Build history of the part. All positions in model axes, mm. A direction names the side the tool comes from. Coordinates: 2 decimals unless noted, no trailing zeros. Loops run counter-clockwise (first coordinate to the right, second up) from the corner with the lowest first, then second, coordinate; pieces in that order, holes last. Notation, with made-up numbers: (55, 89) -> (85, 89) arc R27 cw to (85, 113) -> close; hole circle Ø4 at (69.25, 14.5). An arc over 180 degrees is marked (long way). One line per item, written item: value. Start each with the question number.
Autodesk Inventor part; units mm, degrees
ref_plane "YZ Plane" through (0, 0, 0) normal (1, 0, 0) x (0, 1, 0)
ref_plane "XZ Plane" through (0, 0, 0) normal (0, 1, 0) x (-1, 0, 0)
ref_plane "XY Plane" through (0, 0, 0) normal (0, 0, 1) x (1, 0, 0)
sketch "Esboço1" plane through (0, 0, 0) normal (0, 0, 1) x (1, 0, 0)
  circle A0 centre (0, 0) radius 9
  circle A1 centre (0, 0) radius 11
  point P0 (0, 0)
  dimension "d0" = 2
extrude "Extrusão1" add sketch "Esboço1" along normal blind 5 contours A0 | A1
sketch "Esboço2" plane through (0, 0, 0) normal (0, 0, -1) x (-1, 0, 0)
  circle A0 centre (0, 0) radius 9
  circle A1 centre (0, 0) radius 10
  point P0 (0, 0)
  dimension "d3" = 1
extrude "Extrusão2" add sketch "Esboço2" along normal blind 10
hole "Furo1" at (0, 0, 5) direction (0, 0, -1) diameter 7 depth 8 tip angle 118
properties part number "Corpo Valvula Reguladora de Pressão"
Item 1: Two-plate mould, pull along X, no slides. Class faces 1 (the face through (2, -10, 0)), 2 (the face through (1.341, -3.233, 2.465)), 3 (the face through (2.17, 9.76, -4.93)): +X half, -X half, draft (parallel to the pull), parting line (faces both ways), or undercut.
Item 2: Band-saw the part on D-D, the plane z = -4.25. List the corners of the cut face in (x, y).
Item 3: Drop flat-ended pins along their axis: pin 1 Ø3 at (y, z) = (-4.5, 2) entering from -X; pin 2 Ø8 at (y, z) = (6.5, -4.5) entering from +X; pin 3 Ø8 at (x, z) = (4, -5) entering from -Y. Give the stop position or say it passes through.
Item 4: Band-saw the part on C-C, the plane x = 5.25. List the corners of the cut face in (y, z).
Item 5: Probe probe 1 along Y at (x, z) = (0, -8); probe 2 along Y at (x, z) = (0, 1.15); probe 3 along Z at (x, y) = (2.5, 4). List the from-to ranges inside material, lowest first.
Item 6: Band-saw the part on B-B, the plane y = -3. List the corners of the cut face in (x, z).
Item 7: Tool access for faces 4 (the face through (-2.38, 10.74, 2.46)), 5 (the face through (1.172, -8.923, -4.93)): list every direction of +Z, -Z, +X, -X, +Y, -Y with a clear straight run to the whole face (end or side of a thin tool).
Item 8: Band-saw the part on A-A, the plane x = 0. List the corners of the cut face in (y, z).
Worked out:
1. face 1: draft
1. face 2: undercut
1. face 3: parting line
2. outline: circle Ø20 at (0, 0); hole circle Ø18 at (0, 0)
3. pin 1: stops at x = -10.58
3. pin 2: stops at x = 9.68
3. pin 3: stops at y = -10
4. outline: (-9.67, 0) -> (-8.51, 0) -> (-8.51, -10) -> (-7.31, -10) -> (-7.31, 0) -> (7.31, 0) -> (7.31, -10) -> (8.51, -10) -> (8.51, 0) -> (9.67, 0) -> (9.67, 5) -> (-9.67, 5) -> close
5. probe 1: y = -10 to -9, 9 to 10
5. probe 2: y = -11 to -3.5, 3.5 to 11
5. probe 3: z = 0 to 5
6. outline: (-10.58, 0) -> (-9.54, 0) -> (-9.54, -10) -> (-8.49, -10) -> (-8.49, 0) -> (-1.8, 0) -> (-1.8, 5) -> (-10.58, 5) -> close; (1.8, 0) -> (8.49, 0) -> (8.49, -10) -> (9.54, -10) -> (9.54, 0) -> (10.58, 0) -> (10.58, 5) -> (1.8, 5) -> close
7. face 4: +Z, -Z
7. face 5: -Z
8. outline: (-11, 0) -> (-10, 0) -> (-10, -10) -> (-9, -10) -> (-9, 0) -> (-3.5, 0) -> (-3.5, 5) -> (-11, 5) -> close; (3.5, 0) -> (9, 0) -> (9, -10) -> (10, -10) -> (10, 0) -> (11, 0) -> (11, 5) -> (3.5, 5) -> close
